```python
from build123d import *

# Parameters (mm, degrees)
BOSS_EXTRUDE1_DEPTH      = 165
BOSS_EXTRUDE1_DEPTH_BACK = 35
SKETCH1_R                = 2.5
SKETCH2_W                = 15
SKETCH2_H                = 10
BOSS_EXTRUDE2_DEPTH      = 35
SKETCH3_R                = 5
CUT_EXTRUDE1_DEPTH       = 209.3416665
FILLET1_RADIUS           = 7.5
FILLET1_LENGTH           = 10
FILLET2_R                = 2
SKETCH4_R                = 7.5
BOSS_EXTRUDE3_DEPTH      = 5
FILLET3_R                = 2


with BuildPart() as part:
    # Sketch1 → Boss-Extrude1 (new, two sides: drawn at the far end of the back side and taken through both)
    with BuildSketch(Plane.XY.offset(-BOSS_EXTRUDE1_DEPTH_BACK)):
        with Locations((50, 0)):
            Circle(SKETCH1_R)
    extrude(amount=BOSS_EXTRUDE1_DEPTH + BOSS_EXTRUDE1_DEPTH_BACK)

    # Sketch2 → Boss-Extrude2 (add)
    with BuildSketch(Plane.XY.offset(165)):
        with Locations((50, 0)):
            Rectangle(SKETCH2_W, SKETCH2_H)
    extrude(amount=BOSS_EXTRUDE2_DEPTH)

    # Sketch3 → Cut-Extrude1 (cut, through all)
    with BuildSketch(Plane(origin=(0, 5, 0), x_dir=(1, 0, 0), z_dir=(0, 1, 0))):
        with Locations(Location((50, -190, 0), (0, 0, 270))):
            Circle(SKETCH3_R)
    extrude(amount=-CUT_EXTRUDE1_DEPTH, mode=Mode.SUBTRACT)

    # Fillet1: full round fillet: the end face becomes a half cylinder, R = half its width
    fillet1_face = Plane((50, 0, 200), x_dir=(0, -1, 0), z_dir=(0, 0, 1))  # on the end face: x along it, z out of the body
    fillet1_slab = fillet1_face.offset(-FILLET1_RADIUS / 2) * Box(FILLET1_LENGTH, 2 * FILLET1_RADIUS, FILLET1_RADIUS, mode=Mode.PRIVATE)  # the body's end, R deep
    fillet1_round = Plane((50, 0, 192.5), x_dir=(0, 0, 1), z_dir=(0, -1, 0)) * Cylinder(FILLET1_RADIUS, FILLET1_LENGTH, mode=Mode.PRIVATE)  # its axis R under the face
    add(fillet1_slab - fillet1_round, mode=Mode.SUBTRACT)

    # Fillet2
    fillet2_edges = [part.edges().sort_by_distance(p)[0] for p in [
        (47.5, 0, 165),
    ]]
    fillet(fillet2_edges, radius=FILLET2_R)

    # Sketch4 → Boss-Extrude3 (add)
    with BuildSketch(Plane(origin=(0, 0, -35), x_dir=(-1, 0, 0), z_dir=(0, 0, -1))):
        with Locations((-50, 0)):
            Circle(SKETCH4_R)
    extrude(amount=BOSS_EXTRUDE3_DEPTH)

    # Fillet3
    fillet3_edges = [part.edges().sort_by_distance(p)[0] for p in [
        (47.5, 0, -35),
    ]]
    fillet(fillet3_edges, radius=FILLET3_R)


solid = part.part
```
Source: CAD feature listing. Evaluate the final solid. Frame: model axes, mm. A direction names the side the tool comes from. Give positions to 0.01 mm unless a question says otherwise; leave off trailing zeros. Write each loop counter-clockwise with the first axis right and the second up, starting at its lowest first coordinate (ties: lowest second). Pieces come first, ordered by that corner, then holes. Notation, with made-up numbers: (46, 1) - (85, 1) arc R14 cw to (85, 5) - close; hole circle Ø6 at (-23, 54). An arc over 180 degrees is marked (long way). One line per item, written item: value. Start each with the question number.
Q1. Section query C-C, the plane z = 113. Return the cut outline in (x, y), then the cut area to 3 significant figures.
Q2. Set-up query: faces 1 (the face through (42.846, 2.253, -37.465)), 2 (the face through (46.6, 3.4, 165)), 3 (the face through (50, -5, 182)). Return all of +Z, -Z, +X, -X, +Y, -Y with unobstructed straight access to the full face (end or side cutting, diameter ignored); none if empty.
Q3. Section query A-A, the plane z = 190. Return the cut outline in (x, y), then the cut area to 3 significant figures.
Q4. Section query B-B, the plane y = 0. Return the cut outline in (x, z).
Q5. First-contact query: pin 1 Ø8 at (y, z) = (3.5, 75) entering from +X; pin 2 Ø7.5 at (x, z) = (52, 187.5) entering from -Y; pin 3 Ø1.5 at (x, z) = (45.5, 22.5) entering from -Y; pin 4 Ø4.5 at (x, z) = (53, 181.5) entering from +Y. Flat tips, straight axial feed; report the tip coordinate or a pass-through.
Q6. Material intervals for probe 1 along Z at (x, y) = (49.5, -4.5); probe 2 along X at (y, z) = (-1.75, 190); probe 3 along Z at (x, y) = (46.5, 1.25), sorted ascending. Write a range as from..to.
Answer:
1. outline: circle Ø5 at (50, 0)
1. area: 19.6 mm2
2. face 1: -Z
2. face 2: none
2. face 3: +Z, +X, -X, -Y
3. outline: (42.5, -5) - (45, -5) - (45, 5) - (42.5, 5) - close; (55, -5) - (57.5, -5) - (57.5, 5) - (55, 5) - close
3. area: 50.0 mm2
4. outline: (42.5, -40) - (57.5, -40) - (57.5, -35) - (54.5, -35) arc R2 cw to (52.5, -33) - (52.5, 163) arc R2 cw to (54.5, 165) - (57.5, 165) - (57.5, 192.5) arc R7.5 ccw to (42.5, 192.5) - (42.5, 165) - (45.5, 165) arc R2 cw to (47.5, 163) - (47.5, -33) arc R2 cw to (45.5, -35) - (42.5, -35) - close; hole circle Ø10 at (50, 190)
5. pin 1: stops at x = 52.5
5. pin 2: stops at y = -5
5. pin 3: passes through
5. pin 4: stops at y = 5
6. probe 1: z = -40..-35, 165..185.03, 194.97..199.98
6. probe 2: x = 42.5..45, 55..57.5
6. probe 3: z = -40..-34.84, 164.84..186.43, 193.57..199.13
